Build history of the part. All positions in model axes, mm. A direction names the side the tool comes from. Give positions to 0.01 mm unless a question says otherwise; leave off trailing zeros. Order: outer loops, then holes, each group sorted by start corner. A loop starts at its lowest first (then second) coordinate and runs counter-clockwise, first axis right, second up. Notation, with made-up numbers: (38, 85) -> (74, 85) arc R6 cw to (74, 94) -> close; hole circle Ø4 at (-17, 31.25). An arc over 180 degrees is marked (long way). Write item = value, one per line. Start each with the question number.
from build123d import *

# Parameters (mm, degrees)
F1_W     = 34
F1_H     = 94
F2_DEPTH = 600
F5_W     = 1100
F5_H     = 10
F6_DEPTH = 40.001


with BuildPart() as f2:
    # F1 (on Right) → F2 (new body, symmetric)
    with BuildSketch(Plane.YZ):
        with BuildLine():
            ThreePointArc((-19.2521204937, -49.7380952381), (-18.3734408372, -51.8594155817), (-16.2521204937, -52.7380952381))
            Line((-16.2521204937, -52.7380952381), (17.7478795063, -52.7380952381))
            ThreePointArc((17.7478795063, -52.7380952381), (19.8691998499, -51.8594155817), (20.7478795063, -49.7380952381))
            Line((20.7478795063, -49.7380952381), (20.7478795063, 44.2619047619))
            ThreePointArc((20.7478795063, 44.2619047619), (19.8691998499, 46.3832251055), (17.7478795063, 47.2619047619))
            Line((17.7478795063, 47.2619047619), (-16.2521204937, 47.2619047619))
            ThreePointArc((-16.2521204937, 47.2619047619), (-18.3734408372, 46.3832251055), (-19.2521204937, 44.2619047619))
            Line((-19.2521204937, 44.2619047619), (-19.2521204937, -49.7380952381))
        make_face()
        with Locations((0.7478795063, -2.7380952381)):
            Rectangle(F1_W, F1_H, mode=Mode.SUBTRACT)
    extrude(amount=F2_DEPTH, both=True)


with BuildPart() as f3_1:
    # F3: copy of F2
    add(f2.part)


with BuildPart() as f2_1:
    add(f2.part)

    # F5 (on face) → F6 (cut, through all)
    with BuildSketch(Plane.XZ.offset(19.2521204937)):
        Rectangle(F5_W, F5_H)
    extrude(amount=-F6_DEPTH, mode=Mode.SUBTRACT)


solid = f2_1.part
(1) Mould opens along Y. For faces 1 (the face through (8, 1, 44.262)), 2 (the face through (8, -19.252, 8)), 3 (the face through (-600, -17, 1)) say: released by +Y, released by -Y, zero draft, split by the parting line, or undercut.
(2) Cut at B-B, the plane y = 1. Give the cut face in (x, z).
(3) Wall check: line 1 (Z direction, x = -111, y = 0); line 2 (Y direction, x = 353, z = -33.5); line 3 (Z direction, x = 367, y = 18.5). Give the ranges that are in metal, low to high. Write a range as [from, to].
(4) Cut at A-A, the plane x = -7. Give the cut face in (y, z).
(5) Flat gauge pins, fed straight in: P1, Ø8, axis at y = -10.5, z = -8, coming from the +X side; P2, Ø0.9, axis at x = -228.5, y = 18.5, coming from the -Z side; P3, Ø0.9, axis at x = -167, y = 20, coming from the +Z side; P4, Ø0.9, axis at x = -217, y = -18, coming from the -Z side. Where does each tip first touch, or does it go through?
(6) 3-axis set-ups, long thin cutter, end or side, ignore diameter. For faces 4 (the face through (8, 1, -52.738)), 5 (the face through (8, 17.748, -14)): which of +Z, -Z, +X, -X, +Y, -Y reach the whole face in a straight line?
(7) Cut at C-C, the plane z = 23.5. Give the cut face in (x, y).
Results:
q1.face_1 = undercut
q1.face_2 = released by -Y
q1.face_3 = zero draft
q2.outline = (-600, -52.74) -> (600, -52.74) -> (600, -49.74) -> (-600, -49.74) -> close; (-600, 44.26) -> (600, 44.26) -> (600, 47.26) -> (-600, 47.26) -> close
q3.line_1 = [-52.74, -49.74], [44.26, 47.26]
q3.line_2 = [-19.25, -16.25], [17.75, 20.75]
q3.line_3 = [-52.64, -5], [5, 47.17]
q4.outline = (-19.25, -49.74) arc R3 ccw to (-16.25, -52.74) -> (17.75, -52.74) arc R3 ccw to (20.75, -49.74) -> (20.75, -5) -> (17.75, -5) -> (17.75, -49.74) -> (-16.25, -49.74) -> (-16.25, -5) -> (-19.25, -5) -> close; (-19.25, 5) -> (-16.25, 5) -> (-16.25, 44.26) -> (17.75, 44.26) -> (17.75, 5) -> (20.75, 5) -> (20.75, 44.26) arc R3 ccw to (17.75, 47.26) -> (-16.25, 47.26) arc R3 ccw to (-19.25, 44.26) -> close
q5.P1 = through
q5.P2 = -52.72
q5.P3 = 46.66
q5.P4 = -52.44
q6.face_4 = -Z, +X, -X, +Y, -Y
q6.face_5 = +X, -X
q7.outline = (-600, -19.25) -> (600, -19.25) -> (600, -16.25) -> (-600, -16.25) -> close; (-600, 17.75) -> (600, 17.75) -> (600, 20.75) -> (-600, 20.75) -> close
